```python
from build123d import *

# Parameters (mm, degrees)
SKETCH2_W                = 5
SKETCH2_H                = 7
BOSS_EXTRUDE1_DEPTH      = 40
SKETCH3_R                = 2.05
CUT_EXTRUDE2_DEPTH       = 40
BOSS_EXTRUDE2_DEPTH      = 30
SKETCH7_W                = 4.5
SKETCH7_H                = 2
CUT_EXTRUDE3_DEPTH       = 76.328383431
SKETCH8_W                = 1.7
SKETCH8_H                = 2
CUT_EXTRUDE4_DEPTH       = 73.729741855
SKETCH9_W                = 6.543059906
SKETCH9_H                = 1
BOSS_EXTRUDE3_DEPTH      = 2
SKETCH10_W               = 4.5
SKETCH10_H               = 75
CUT_EXTRUDE5_DEPTH       = 1.5
SKETCH13_W               = 2.8
SKETCH13_H               = 2
CUT_EXTRUDE7_DEPTH       = 1.5
SKETCH15_W               = 1.5
SKETCH15_H               = 2
CUT_EXTRUDE8_DEPTH       = 18.5
SKETCH16_R               = 1.25
CUT_EXTRUDE9_DEPTH       = 3.5
SKETCH17_R               = 1.25
CUT_EXTRUDE10_DEPTH      = 3.5
SKETCH18_W               = 22.143059906
SKETCH18_H               = 3
BOSS_EXTRUDE4_DEPTH      = 15.5
BOSS_EXTRUDE5_DEPTH      = 13
BOSS_EXTRUDE5_DEPTH_BACK = 2
SKETCH19_W               = 13.83663494
SKETCH19_H               = 3
BOSS_EXTRUDE6_DEPTH      = 2.5
BOSS_EXTRUDE8_DEPTH      = 2.5
BOSS_EXTRUDE9_DEPTH      = 4.2
BOSS_EXTRUDE10_DEPTH     = 4.2
SKETCH25_R               = 2.05
CUT_EXTRUDE12_DEPTH      = 3.5
CUT_EXTRUDE13_DEPTH      = 71.528016285
CUT_EXTRUDE14_DEPTH      = 71.528016285


with BuildPart() as part:
    # Sketch2 → Boss-Extrude1 (new body)
    with BuildSketch(Plane(origin=(0, 0, 0), x_dir=(1, 0, 0), z_dir=(0, 1, 0))):
        Polygon((9.921548121, -11.656419986), (5.768335638, 3.843580014), (5.768335638, 1.343580014), (3.850018168, 1.343580014), (7.33335767, -11.656419986), align=None)
        Polygon((5.768335638, 3.843580014), (-8.068299302, 3.843580014), (-5.653484736, 3.196532402), (-6.149981832, 1.343580014), (3.850018168, 1.343580014), (3.353521072, 3.196532402), align=None)
        Polygon((-8.068299302, 1.343580014), (-8.068299302, 3.843580014), (-12.221511785, -11.656419986), (-9.633321334, -11.656419986), (-6.149981832, 1.343580014), align=None)
        Polygon((5.768335638, 1.343580014), (5.768335638, 3.843580014), (3.353521072, 3.196532402), (3.850018168, 1.343580014), align=None)
        Polygon((-5.653484736, 3.196532402), (-8.068299302, 3.843580014), (-8.068299302, 1.343580014), (-6.149981832, 1.343580014), align=None)
        Polygon((-9.806697219, -12.303467598), (-12.221511785, -11.656419986), (-12.221511785, -14.156419986), (-9.421511785, -14.156419986), (-4.421511785, -14.156419986), (-4.421511785, -11.656419986), (-9.633321334, -11.656419986), align=None)
        Polygon((-9.633321334, -11.656419986), (-12.221511785, -11.656419986), (-9.806697219, -12.303467598), align=None)
        Polygon((7.506733555, -12.303467598), (9.921548121, -11.656419986), (7.33335767, -11.656419986), align=None)
        Polygon((9.921548121, -14.156419986), (9.921548121, -11.656419986), (7.506733555, -12.303467598), (7.33335767, -11.656419986), (2.121548121, -11.656419986), (2.121548121, -14.156419986), (7.121548121, -14.156419986), align=None)
        with Locations((4.621548121, -17.656419986)):
            Rectangle(SKETCH2_W, SKETCH2_H)
        with Locations((-6.921511785, -17.656419986)):
            Rectangle(SKETCH2_W, SKETCH2_H)
    extrude(amount=BOSS_EXTRUDE1_DEPTH)

    # Sketch3 → Cut-Extrude2 (cut)
    with BuildSketch(Plane.ZY.offset(9.421511785)):
        with Locations((17.656419986, 33)):
            Circle(SKETCH3_R)
        with Locations((17.656419986, 7)):
            Circle(SKETCH3_R)
    extrude(amount=-CUT_EXTRUDE2_DEPTH, mode=Mode.SUBTRACT)

    # Sketch4 → Boss-Extrude2 (add)
    with BuildSketch(Plane(origin=(0, 40, 0), x_dir=(1, 0, 0), z_dir=(0, 1, 0))):
        Polygon((-4.421511785, -11.656419986), (-9.633321334, -11.656419986), (-6.149981832, 1.343580014), (3.850018168, 1.343580014), (7.33335767, -11.656419986), (2.121548121, -11.656419986), (2.121548121, -14.156419986), (7.121548121, -14.156419986), (9.921548121, -14.156419986), (9.921548121, -11.656419986), (5.768335638, 3.843580014), (-8.068299302, 3.843580014), (-12.221511785, -11.656419986), (-12.221511785, -14.156419986), (-9.421511785, -14.156419986), (-4.421511785, -14.156419986), align=None)
    extrude(amount=BOSS_EXTRUDE2_DEPTH)

    # Sketch7 → Cut-Extrude3 (cut, through all)
    with BuildSketch(Plane(origin=(0, 0, -3.843580014), x_dir=(-1, 0, 0), z_dir=(0, 0, -1))):
        with Locations((3.241664362, 39)):
            Rectangle(SKETCH7_W, SKETCH7_H)
    extrude(amount=-CUT_EXTRUDE3_DEPTH, mode=Mode.SUBTRACT)

    # Sketch8 → Cut-Extrude4 (cut, through all)
    with BuildSketch(Plane(origin=(0, 0, 11.656419986), x_dir=(-1, 0, 0), z_dir=(0, 0, -1))):
        with Locations((5.271511785, 4.2)):
            Rectangle(SKETCH8_W, SKETCH8_H)
    extrude(amount=-CUT_EXTRUDE4_DEPTH, mode=Mode.SUBTRACT)

    # Sketch9 → Boss-Extrude3 (add)
    with BuildSketch(Plane(origin=(0, 70, 0), x_dir=(1, 0, 0), z_dir=(0, 1, 0))):
        Polygon((7.33335767, -11.656419986), (2.121548121, -11.656419986), (2.121548121, -12.656419986), (8.636583042, -12.656419986), (4.617345156, 2.343580014), (-6.91730882, 2.343580014), (-10.936546706, -12.656419986), (-4.421511785, -12.656419986), (-4.421511785, -11.656419986), (-9.633321334, -11.656419986), (-6.149981832, 1.343580014), (3.850018168, 1.343580014), align=None)
        with Locations((-1.149981832, -12.156419986)):
            Rectangle(SKETCH9_W, SKETCH9_H)
    extrude(amount=BOSS_EXTRUDE3_DEPTH)

    # Sketch10 → Cut-Extrude5 (cut)
    with BuildSketch(Plane(origin=(0, 0, -3.843580014), x_dir=(-1, 0, 0), z_dir=(0, 0, -1))):
        with Locations((3.241664362, 77.5)):
            Rectangle(SKETCH10_W, SKETCH10_H)
    extrude(amount=-CUT_EXTRUDE5_DEPTH, mode=Mode.SUBTRACT)

    # Sketch13 → Cut-Extrude7 (cut)
    with BuildSketch(Plane(origin=(0, 0, -2.343580014), x_dir=(-1, 0, 0), z_dir=(0, 0, -1))):
        with Locations((6.891664362, 41)):
            Rectangle(SKETCH13_W, SKETCH13_H)
    extrude(amount=CUT_EXTRUDE7_DEPTH, mode=Mode.SUBTRACT)

    # Sketch15 → Cut-Extrude8 (cut, along a direction that is not the sketch's normal)
    with BuildSketch(Plane(origin=(0, 0, -3.843580014), x_dir=(-1, 0, 0), z_dir=(0, 0, -1))):
        with Locations((7.318299302, 41)):
            Rectangle(SKETCH15_W, SKETCH15_H)
    extrude(amount=-CUT_EXTRUDE8_DEPTH, dir=(0.25881904510252474, 0, -0.9659258262890672), mode=Mode.SUBTRACT)

    # Sketch16 → Cut-Extrude9 (cut, along a direction that is not the sketch's normal)
    with BuildSketch(Plane.XY.offset(14.156419986)):
        with Locations((-7.421511785, 50)):
            Circle(SKETCH16_R)
    extrude(amount=-CUT_EXTRUDE9_DEPTH, dir=(-0.2588190451025246, 0, 0.9659258262890672), mode=Mode.SUBTRACT)

    # Sketch17 → Cut-Extrude10 (cut, along a direction that is not the sketch's normal)
    with BuildSketch(Plane.XY.offset(14.156419986)):
        with Locations((5.121548121, 50)):
            Circle(SKETCH17_R)
    extrude(amount=-CUT_EXTRUDE10_DEPTH, dir=(0.25881904510251796, 0, 0.9659258262890691), mode=Mode.SUBTRACT)

    # Sketch18 → Boss-Extrude4 (add)
    with BuildSketch(Plane(origin=(0, 0, 11.656419986), x_dir=(-1, 0, 0), z_dir=(0, 0, -1))):
        with Locations((1.149981832, 68.5)):
            Rectangle(SKETCH18_W, SKETCH18_H)
    extrude(amount=-BOSS_EXTRUDE4_DEPTH)

    # Sketch19 → Boss-Extrude5 (add, two sides: drawn at the far end of the back side and taken through both)
    with BuildSketch(Plane(origin=(0, 0, -3.843580014), x_dir=(-1, 0, 0), z_dir=(0, 0, -1)).offset(-BOSS_EXTRUDE5_DEPTH_BACK)):
        with Locations((1.149981832, 68.5)):
            Rectangle(SKETCH19_W, SKETCH19_H)
    extrude(amount=BOSS_EXTRUDE5_DEPTH + BOSS_EXTRUDE5_DEPTH_BACK)

    # Sketch21 → Boss-Extrude6 (add)
    with BuildSketch(Plane.ZY.offset(12.221511785)):
        Polygon((27.156419986, 67), (14.156419986, 53), (14.156419986, 67), align=None)
    extrude(amount=-BOSS_EXTRUDE6_DEPTH)

    # Sketch22 → Boss-Extrude8 (add)
    with BuildSketch(Plane(origin=(9.921548121, 0, 0), x_dir=(0, 0, -1), z_dir=(1, 0, 0))):
        Polygon((-27.156419986, 67), (-14.156419986, 67), (-14.156419986, 53), align=None)
    extrude(amount=-BOSS_EXTRUDE8_DEPTH)

    # Sketch23 → Boss-Extrude9 (add)
    with BuildSketch(Plane(origin=(9.921548121, 0, 0), x_dir=(0, 0, -1), z_dir=(1, 0, 0))):
        Polygon((-11.656419986, 70), (-11.656419986, 53), (16.843580014, 67), (16.843580014, 70), align=None)
    extrude(amount=-BOSS_EXTRUDE9_DEPTH)

    # Sketch24 → Boss-Extrude10 (add)
    with BuildSketch(Plane.ZY.offset(12.221511785)):
        Polygon((11.656419986, 70), (-16.843580014, 70), (-16.843580014, 67), (11.656419986, 53), align=None)
    extrude(amount=-BOSS_EXTRUDE10_DEPTH)

    # Sketch25 → Cut-Extrude12 (cut)
    with BuildSketch(Plane(origin=(0, 70, 0), x_dir=(1, 0, 0), z_dir=(0, 1, 0))):
        with Locations(Location((-1.149981694, 10.343580014, 0), (0, 0, 270))):
            Circle(SKETCH25_R)
        with Locations(Location((-1.149981723, -20.656419986, 0), (0, 0, 270))):
            Circle(SKETCH25_R)
    extrude(amount=-CUT_EXTRUDE12_DEPTH, mode=Mode.SUBTRACT)

    # Sketch26 → Cut-Extrude13 (cut, through all, along a direction that is not the sketch's normal)
    with BuildSketch(Plane(origin=(0, 47.309855268, 23.239928904), x_dir=(-1, 0, 0), z_dir=(-4.742047126241555e-14, -0.8975543264374147, -0.4409038796534669))):
        Polygon((-5.721548121, 12.905635433), (-7.33335767, 12.905635433), (-5.721548121, 19.607575306), align=None)
        Polygon((8.021511785, 12.905635433), (8.021511785, 19.607575306), (9.633321334, 12.905635433), align=None)
    extrude(amount=-CUT_EXTRUDE13_DEPTH, dir=(0, -1, 0), mode=Mode.SUBTRACT)

    # Sketch27 → Cut-Extrude14 (cut, through all, along a direction that is not the sketch's normal)
    with BuildSketch(Plane(origin=(0, 47.309855268, 23.239928904), x_dir=(-1, 0, 0), z_dir=(0, -0.8975543264374147, -0.440903879653467))):
        Polygon((12.221511785, 12.905635433), (10.521511785, 44.658588051), (12.221511785, 44.658588051), align=None)
        Polygon((-9.921548121, 12.905635433), (-9.921548121, 44.658588051), (-8.221548121, 44.658588051), align=None)
    extrude(amount=-CUT_EXTRUDE14_DEPTH, dir=(0, -1, 0), mode=Mode.SUBTRACT)


solid = part.part
```
Check sheet for the modelled part. Datum: model origin and axes. Units: mm. A direction names the side the tool comes from. Round coordinates to 2 decimals unless told otherwise and drop trailing zeros. Order: outer loops, then holes, each group sorted by start corner. A loop starts at its lowest first (then second) coordinate and runs counter-clockwise, first axis right, second up.
1) Go/stop test with flat-tipped pins: pin 1 Ø3 at (y, z) = (35.5, 18) entering from -X; pin 2 Ø1.5 at (y, z) = (28, 15) entering from +X; pin 3 Ø11 at (x, z) = (-0.5, -13) entering from -Y; pin 4 Ø3.5 at (x, z) = (-1.15, 20.66) entering from +Y. Record where each tip stops, or that it passes through.
2) Tool access check on faces 4 (the flat face through (-1, 71, -2.344)), 5 (the flat face through (7.122, 20, 18)), 6 (the flat face through (-9.422, 20, 18)), 7 (the flat face through (-1, 35, -1.344)). Record the directions out of +Z, -Z, +X, -X, +Y, -Y that give a thin tool (end or side, any length) a straight path to the whole face; none if there is none.
3) Scan lines: line 1 (Z direction, x = 3.5, y = 20); line 2 (Y direction, x = 4, z = 14.5); line 3 (X direction, y = 20.5, z = 15). Record each from-to range of solid material in increasing order.
4) Section check B-B (z = 10.5). Record the boundary of the cut face in (x, y), and give its area (3 significant figures).
5) Section check D-D (x = -2.25). Record the boundary of the cut face in (y, z), and give its area (3 significant figures).
6) Section check A-A (y = 7). Record the boundary of the cut face in (x, z).
7) Section check C-C (y = 19.5). Record the boundary of the cut face in (x, z), and give its area (3 significant figures).
8) Mould release check, pull along Y, two halves, no side actions. Record for faces 1 (the flat face through (8.689, 59.902, 20.565)), 2 (the flat face through (-5, 5.2, 20)), 3 (the flat face through (-4.422, 21, 16)): +Y half, -Y half, draft (parallel to the pull), parting line (faces both ways), or undercut.
Result:
1. pin 1: stops at x = -9.42
1. pin 2: stops at x = 7.12
1. pin 3: stops at y = 67
1. pin 4: passes through
2. face 4: -Z, +X, -X, +Y
2. face 5: +Z, +X, -Y
2. face 6: +Z, -X, -Y
2. face 7: +Y, -Y
3. line 1: z = -3.84 to -1.34, 11.66 to 21.16
3. line 2: y = 0 to 40, 67 to 70
3. line 3: x = -9.42 to -4.42, 2.12 to 7.12
4. outline: (-12.15, 53.57) - (-11.91, 53.57) - (-11.91, 42) - (-10.41, 42) - (-10.41, 40) - (-11.91, 40) - (-11.91, 0) - (-9.32, 0) - (-9.32, 72) - (-10.36, 72) - (-10.36, 70) - (-12.15, 70) - close; (7.02, 0) - (9.61, 0) - (9.61, 53.57) - (9.85, 53.57) - (9.85, 70) - (8.06, 70) - (8.06, 72) - (7.02, 72) - close
4. area: 371 mm2
5. outline: (0, -3.84) - (38, -3.84) - (38, -1.34) - (0, -1.34) - close; (40, -2.34) - (67, -2.34) - (67, -8.61) - (70, -8.61) - (70, -2.34) - (72, -2.34) - (72, -1.34) - (40, -1.34) - close; (67, -16.84) - (70, -16.84) - (70, -12.07) - (67, -12.07) - close; (67, 11.66) - (72, 11.66) - (72, 12.66) - (70, 12.66) - (70, 18.93) - (67, 18.93) - close; (67, 22.39) - (70, 22.39) - (70, 27.16) - (67, 27.16) - close
5. area: 198 mm2
6. outline: (-12.22, 11.66) - (-8.07, -3.84) - (5.77, -3.84) - (9.92, 11.66) - (9.92, 14.16) - (7.12, 14.16) - (7.12, 15.61) - (2.12, 15.61) - (2.12, 11.66) - (7.33, 11.66) - (3.85, -1.34) - (-6.15, -1.34) - (-9.63, 11.66) - (-4.42, 11.66) - (-4.42, 15.61) - (-9.42, 15.61) - (-9.42, 14.16) - (-12.22, 14.16) - close; (-9.42, 19.71) - (-4.42, 19.71) - (-4.42, 21.16) - (-9.42, 21.16) - close; (2.12, 19.71) - (7.12, 19.71) - (7.12, 21.16) - (2.12, 21.16) - close
7. outline: (-12.22, 11.66) - (-8.07, -3.84) - (5.77, -3.84) - (9.92, 11.66) - (9.92, 14.16) - (7.12, 14.16) - (7.12, 21.16) - (2.12, 21.16) - (2.12, 11.66) - (7.33, 11.66) - (3.85, -1.34) - (-6.15, -1.34) - (-9.63, 11.66) - (-4.42, 11.66) - (-4.42, 21.16) - (-9.42, 21.16) - (-9.42, 14.16) - (-12.22, 14.16) - close
7. area: 213 mm2
8. face 1: -Y half
8. face 2: undercut
8. face 3: draft
